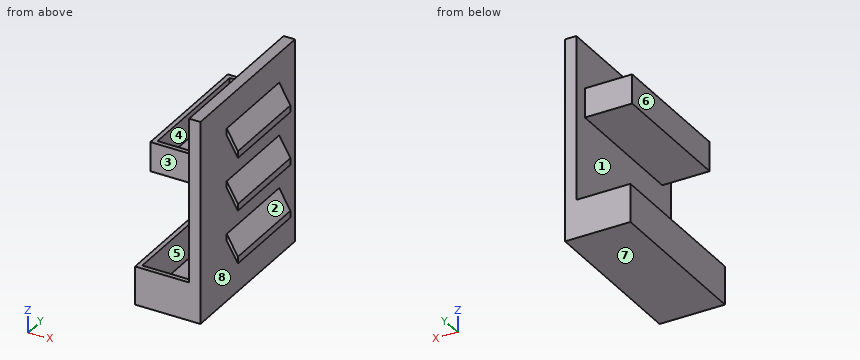
```python
from build123d import *

# Parameters (mm, degrees)
F1_DEPTH  = 90
F2_DEPTH  = 17
F0_W      = 22
F0_H      = 68
F3_DEPTH  = 2
F6_DEPTH  = 13
F5_W      = 19
F5_H      = 55
F7_DEPTH  = 2
F10_DEPTH = 20


with BuildPart() as f1:
    # F0 (on Top) → F1 (new body)
    with BuildSketch(Plane.XY):
        Polygon((2.5, -36), (2.5, 36), (-2.5, 36), (-2.5, 34), (-2.5, -34), (-2.5, -36), align=None)
    extrude(amount=F1_DEPTH)

    # F0 (on Top) → F2 (join)
    with BuildSketch(Plane.XY):
        Polygon((-2.5, 34), (-2.5, 36), (-26.5, 36), (-26.5, -36), (-2.5, -36), (-2.5, -34), (-24.5, -34), (-24.5, 34), align=None)
    extrude(amount=F2_DEPTH)

    # F0 (on Top) → F3 (join)
    with BuildSketch(Plane.XY):
        with Locations((-13.5, 0)):
            Rectangle(F0_W, F0_H)
    extrude(amount=F3_DEPTH)

    # F5 (on offset) → F6 (join)
    with BuildSketch(Plane.XY.offset(57)):
        Polygon((-2.5, 27.5), (-2.5, 29.5), (-23.5, 29.5), (-23.5, -29.5), (-2.5, -29.5), (-2.5, -27.5), (-21.5, -27.5), (-21.5, 27.5), align=None)
    extrude(amount=F6_DEPTH)

    # F5 (on offset) → F7 (join)
    with BuildSketch(Plane.XY.offset(57)):
        with Locations((-12, 0)):
            Rectangle(F5_W, F5_H)
    extrude(amount=F7_DEPTH)

    # F9 (on offset) → F10 (join, symmetric)
    with BuildSketch(Plane.XZ.offset(-4)):
        Polygon((7.5, 68.2301041718), (2.5, 76.8903582096), (2.5, 73.8903582096), (7.5, 65.2301041718), align=None)
        Polygon((7.5, 44.7301041718), (2.5, 53.3903582096), (2.5, 50.3903582096), (7.5, 41.7301041718), align=None)
        Polygon((7.5, 21.2301041718), (2.5, 29.8903582096), (2.5, 26.8903582096), (7.5, 18.2301041718), align=None)
    extrude(amount=F10_DEPTH, both=True)


solid = f1.part
```
Here's how the part is built. I have some questions about the finished solid (model axes, mm). Face numbers are marked on the shaded views. A direction names the side the tool comes from. Give positions to 0.01 mm unless a question says otherwise; leave off trailing zeros. Loops run counter-clockwise (first coordinate to the right, second up) from the corner with the lowest first, then second, coordinate; pieces in that order, holes last. Notation, with made-up numbers: M 6,15.5 L 32,15.5 A25 ccw 32,41.5 Z; hole C 9,2.5 d9. An arc over 180 degrees is marked long. Use one line per item in the form item = value. Start each with the question number.
Q1. Which directions (+Z, -Z, +X, -X, +Y, -Y) give clear straight access to the entire face, cutting with the end or side of a thin tool? Please do the marked faces 1, 2, 3 and 4.
Q2. Thinking about a two-plate mould opening in X: for the marked faces 5, 6, 7 and 8, which applies, +X half, -X half, draft (parallel to the pull), parting line (faces both ways), or undercut?
Q3. If we section it at B-B (z = 16): Write out the boundary of the cut face in (x, y), then the cut area to 3 significant figures.
Q4. I need wall thicknesses on line 1 along Z through (x, y) = (-6.5, 0); line 2 along Y through (x, z) = (-21.5, 11.5); line 3 along Z through (x, y) = (-22, -11). Which ranges of each line are inside material? Lowest first, please.
Q5. Will these pins go through, and if not, where does the flat tip stop? pin 1 Ø12 at (x, y) = (-16.5, 7) entering from +Z; pin 2 Ø10 at (y, z) = (-16, 40.5) entering from -X; pin 3 Ø1.5 at (x, z) = (5.5, 25) entering from -Y.
Q6. If we section it at A-A (x = -14.5): Write out the boundary of the cut face in (y, z).
Q7. If we section it at C-C (x = 3.5): Write out the boundary of the cut face in (y, z).
Q8. If we section it at D-D (y = 23): Write out the boundary of the cut face in (x, z).
Taken from the geometry:
q1.face_1 = none
q1.face_2 = +X, +Y, -Y
q1.face_3 = +Z, -X, -Y
q1.face_4 = +Z
q2.face_5 = undercut
q2.face_6 = -X half
q2.face_7 = draft
q2.face_8 = undercut
q3.outline = M -26.5,-36 L 2.5,-36 L 2.5,36 L -26.5,36 Z; hole M -24.5,-34 L -2.5,-34 L -2.5,34 L -24.5,34 Z
q3.area = 592 mm^2
q4.line_1 = 0 to 2, 57 to 59
q4.line_2 = -36 to -34, 34 to 36
q4.line_3 = 0 to 2, 57 to 70
q5.pin_1 = 70
q5.pin_2 = -2.5
q5.pin_3 = -16
q6.outline = M -36,0 L 36,0 L 36,17 L 34,17 L 34,2 L -34,2 L -34,17 L -36,17 Z; M -29.5,57 L 29.5,57 L 29.5,70 L 27.5,70 L 27.5,59 L -27.5,59 L -27.5,70 L -29.5,70 Z
q7.outline = M -16,25.16 L 24,25.16 L 24,28.16 L -16,28.16 Z; M -16,48.66 L 24,48.66 L 24,51.66 L -16,51.66 Z; M -16,72.16 L 24,72.16 L 24,75.16 L -16,75.16 Z
q8.outline = M -26.5,0 L 2.5,0 L 2.5,26.89 L 7.5,18.23 L 7.5,21.23 L 2.5,29.89 L 2.5,50.39 L 7.5,41.73 L 7.5,44.73 L 2.5,53.39 L 2.5,73.89 L 7.5,65.23 L 7.5,68.23 L 2.5,76.89 L 2.5,90 L -2.5,90 L -2.5,59 L -21.5,59 L -21.5,70 L -23.5,70 L -23.5,57 L -2.5,57 L -2.5,2 L -24.5,2 L -24.5,17 L -26.5,17 Z
